```python
from build123d import *

# Parameters (mm, degrees)
F1_DEPTH  = 10
F2_W      = 2
F2_H      = 10
F3_DEPTH  = 25
F4_DEPTH  = 44.001
F6_DEPTH  = 41.001
F9_DEPTH  = 3
F10_SIZE  = 2.99999
F12_DEPTH = 3
F13_SIZE  = 2.99999
F16_D     = 2
F17_D     = 2


# Not quite as in the source:
# - a fillet or chamfer is up to 0.001 mm smaller than in the source, because OpenCascade refuses the exact size
# - a feature of the source that left no trace in its solid (it failed there, or was rolled back) is left out


with BuildPart() as f1:
    # F0 (on Top) → F1 (new body)
    with BuildSketch(Plane.XY):
        Polygon((-22, -19.5), (-20, -19.5), (-20, 19.5), (20, 19.5), (20, 21.5), (-22, 21.5), align=None)
        Polygon((20, 19.5), (20, -19.5), (-20, -19.5), (-22, -19.5), (-22, -21.5), (22, -21.5), (22, 21.5), (20, 21.5), align=None)
    extrude(amount=-F1_DEPTH)

    # F2 (on face) → F3 (cut)
    with BuildSketch(Plane(origin=(-22, 0, 0), x_dir=(0, -1, 0), z_dir=(-1, 0, 0))):
        with Locations((20.5, -5)):
            Rectangle(F2_W, F2_H)
        Polygon((13.5, -10), (18.9169048105, -10), (13.5, -0.9718253158), align=None)
    extrude(amount=-F3_DEPTH, mode=Mode.SUBTRACT)

    # F2 (on face) → F4 (cut, through all)
    with BuildSketch(Plane(origin=(-22, 0, 0), x_dir=(0, -1, 0), z_dir=(-1, 0, 0))):
        Polygon((19.5, 0), (13.5, 0), (19.5, -10), align=None)
        with Locations((20.5, -5)):
            Rectangle(F2_W, F2_H)
    extrude(amount=-F4_DEPTH, mode=Mode.SUBTRACT)

    # F5 (on face) → F6 (cut, through all)
    with BuildSketch(Plane(origin=(0, 21.5, 0), x_dir=(-1, 0, 0), z_dir=(0, 1, 0))):
        Polygon((-14, -0.9077913453), (-20, -10), (-14, -10), align=None)
        Polygon((-22, -10), (-20, -10), (-20, -9.0922086547), (-14, 0), (-22, 0), align=None)
    extrude(amount=-F6_DEPTH, mode=Mode.SUBTRACT)

    # F8 (on face) → F9 (join)
    with BuildSketch(Plane(origin=(0, 21.5, 0), x_dir=(-1, 0, 0), z_dir=(0, 1, 0))):
        Polygon((-14, -10), (-9, -10), (-9, 0), (-14, 0), (-20, -9.0922086547), (-20, -10), (-14, -0.9077913453), align=None)
    extrude(amount=F9_DEPTH)

    # F10 (size 3 in the source; OpenCascade refuses exactly that, so slightly less here)
    f10_edges = [f1.edges().sort_by_distance(p)[0] for p in [
        (9, 24.5, -5),
    ]]
    chamfer(f10_edges, length=F10_SIZE)

    # F11 (on face) → F12 (join)
    with BuildSketch(Plane(origin=(-22, 0, 0), x_dir=(0, -1, 0), z_dir=(-1, 0, 0))):
        Polygon((13.5, 0), (8.5, 0), (8.5, -10), (13.5, -10), (13.5, -0.9718253158), (18.9169048105, -10), (19.5, -10), align=None)
    extrude(amount=F12_DEPTH)

    # F13 (size 3 in the source; OpenCascade refuses exactly that, so slightly less here)
    f13_edges = [f1.edges().sort_by_distance(p)[0] for p in [
        (-25, -8.5, -5),
    ]]
    chamfer(f13_edges, length=F13_SIZE)

    # F16 (through all)
    with Locations(Plane(origin=(-22, 0, 0), x_dir=(0, -1, 0), z_dir=(-1, 0, 0))):
        with Locations((-6.5, -3), (3.5, -3), (-16.5, -3)):
            Hole(F16_D / 2)

    # F17 (through all)
    with Locations(Plane(origin=(0, 21.5, 0), x_dir=(-1, 0, 0), z_dir=(0, 1, 0))):
        with Locations((-3.5, -3), (6.5, -3), (16.5, -3)):
            Hole(F17_D / 2)


solid = f1.part
```
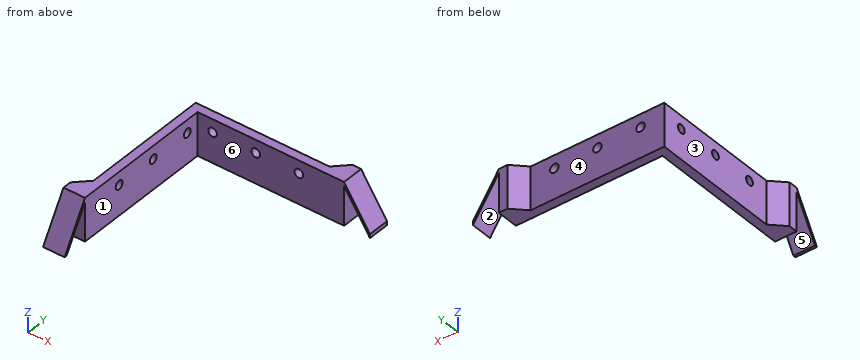
Verification items for the finished model (mm, model axes). Face numbers are marked on the shaded views. A direction names the side the tool comes from. Coordinates: 2 decimals unless noted, no trailing zeros. Write each loop counter-clockwise with the first axis right and the second up, starting at its lowest first coordinate (ties: lowest second). Pieces come first, ordered by that corner, then holes. Notation, with made-up numbers: M 89,9.5 L 105,9.5 A18 ccw 105,35.5 Z; hole C 68.5,70 d4. An arc over 180 degrees is marked long. Answer as a JSON object with one key per item and string values. Group by question number.
(1) Material ranges on line 1 (Z direction, x = -21.5, y = 16.5); line 2 (Y direction, x = 12, z = -3.75); line 3 (X direction, y = 13, z = -3.5), recorded low to high.
(2) Cross-section at C-C, the plane z = -7.25. State how many separate pieces and enclosed holes the cut face has, and give its area (3 significant figures).
(3) Cross-section at A-A, the plane y = 6.5. Record the cut outline in (x, z), and give its area (3 significant figures).
(4) Gauge pin test, flat ends, axial feed: pin 1 (5 mm diameter, centred on x = 9, z = -7, fed in from -Y); pin 2 (5 mm diameter, centred on y = -8, z = -6.5, fed in from +X); pin 3 (2.5 mm diameter, centred on x = -6.5, z = -3, fed in from +Y). Record the tip position at first contact, or that the pin passes through.
(5) Tool access check on the marked faces 1, 2 and 3. Record the directions out of +Z, -Z, +X, -X, +Y, -Y that give a thin tool (end or side, any length) a straight path to the whole face; none if there is none.
(6) Cross-section at B-B, the plane x = -16.5. Record the cut outline in (y, z), and give its area (3 significant figures).
(7) Cross-section at D-D, the plane x = -4. Record the cut outline in (y, z).
(8) Release check for a two-part mould opening along Y. For the marked faces 4, 5 and 6 record: +Y half, -Y half, draft (parallel to the pull), parting line (faces both ways), or undercut.
Reply:
{
 "1": {"line 1": "-10 to -4, -2 to 0", "line 2": "19.5 to 24.5", "line 3": "-22 to -20"},
 "2": {"separate pieces": "3", "enclosed holes": "0", "area": "165 mm²"},
 "3": {"outline": "M -22,-10 L -20,-10 L -20,-4 L -22,-4 Z; M -22,-2 L -20,-2 L -20,0 L -22,0 Z", "area": "16.0 mm²"},
 "4": {"pin 1": "y = 19.5", "pin 2": "x = -20", "pin 3": "y = 21.5"},
 "5": {"face 1": "+Z, -Z, +X, -Y", "face 2": "-Z, +Y, -Y", "face 3": "+Z, -Z, -X, +Y"},
 "6": {"outline": "M 19.5,-10 L 21.5,-10 L 21.5,-4 L 19.5,-4 Z; M 19.5,-2 L 21.5,-2 L 21.5,0 L 19.5,0 Z", "area": "16.0 mm²"},
 "7": {"outline": "M 19.5,-10 L 21.5,-10 L 21.5,0 L 19.5,0 Z"},
 "8": {"face 4": "+Y half", "face 5": "undercut", "face 6": "-Y half"}
}
